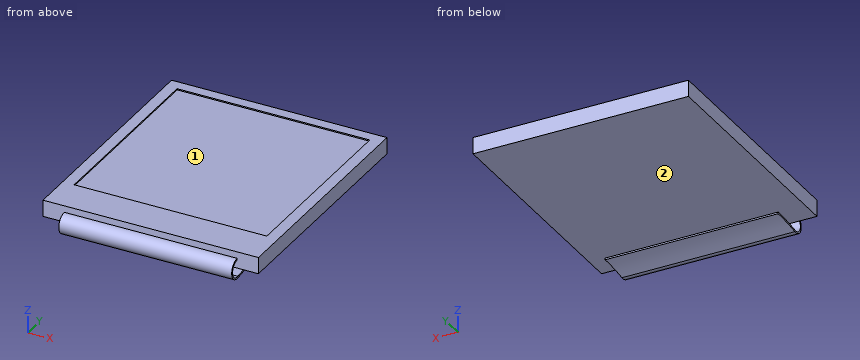
```python
from build123d import *

# Parameters (mm, degrees)
SKETCH001_W     = 26.16
SKETCH001_H     = 29.22
PAD001_DEPTH    = 2
SKETCH003_W     = 23.4
SKETCH003_H     = 23.4
POCKET001_DEPTH = 0.151
PAD002_DEPTH    = 10.5


with BuildPart() as part:
    # Sketch001 → Pad001 (new body)
    with BuildSketch(Plane.XY.offset(2.8)):
        Rectangle(SKETCH001_W, SKETCH001_H)
    extrude(amount=-PAD001_DEPTH)

    # Sketch003 → Pocket001 (cut, through all)
    with BuildSketch(Plane.XY.offset(2.65)):
        with Locations((0, 1.58)):
            Rectangle(SKETCH003_W, SKETCH003_H)
    extrude(amount=POCKET001_DEPTH, mode=Mode.SUBTRACT)

    # Sketch004 → Pad002 (join, symmetric)
    with BuildSketch(Plane.YZ):
        with BuildLine():
            ThreePointArc((-14.61, 2), (-15.856499, 0.656513), (-14.423549, -0.486016))
            ThreePointArc((-10.61, -0.2), (-12.52213, -0.271604), (-14.423549, -0.486016))
            Line((-10.61, 0), (-10.61, -0.2))
            ThreePointArc((-10.61, 0), (-12.537088, -0.072164), (-14.453381, -0.288254))
            ThreePointArc((-14.61, 1.8), (-15.657059, 0.671471), (-14.453381, -0.288254))
            Line((-14.61, 2), (-14.61, 1.8))
        make_face()
    extrude(amount=PAD002_DEPTH, both=True)


solid = part.part
```
Geometry: final body of the model. Coordinates: model frame, mm. Face numbers are marked on the shaded views. Coordinates: 2 decimals unless noted, no trailing zeros. Write each loop counter-clockwise with the first axis right and the second up, starting at its lowest first coordinate (ties: lowest second). Pieces come first, ordered by that corner, then holes. Notation, with made-up numbers: M -25.75,53.25 L 27.25,53.25 A21 ccw 27.25,76.25 Z; hole C 58.25,-28 d6. An arc over 180 degrees is marked long. Use CSV: the item, a comma, the result in double quotes. Start each with the question number.
1. Cut plane D-D on y = 8. Return the cut outline in (x, z), plus the area to 3 significant figures.
2. Mould query, pull axis X, two halves, no side actions, for the marked faces 1 and 2. Classes: pulls with the +X half, pulls with the -X half, needs draft (parallel to the pull), parting line crosses it, or undercut.
3. Cut plane C-C on x = -6.75. Return the cut outline in (y, z), plus the area to 3 significant figures.
4. Cut plane A-A on z = 1.35. Return the cut outline in (x, y), plus the area to 3 significant figures.
5. First-contact query: P1, Ø0.6, axis at x = 3.5, z = 2, coming from the -Y side; P2, Ø10, axis at x = -6.5, y = 1.5, coming from the -Z side; P3, Ø7, axis at x = -5.5, y = 5.5, coming from the +Z side; P4, Ø6, axis at x = -3, y = 10.5, coming from the +Z side. Flat tips, straight axial feed; report the tip coordinate or a pass-through.
6. Cut plane B-B on y = -12.5. Return the cut outline in (x, z), plus the area to 3 significant figures.
7. Ray query, probe 1 along Z at (x, y) = (-11.5, -13.5); probe 2 along Z at (x, y) = (10.75, 2.5); probe 3 along Y at (x, z) = (-11.25, 1.6). Return the intervals inside material, ascending.
Entries:
1,outline,"M -13.08,0.8 L 13.08,0.8 L 13.08,2.8 L 11.7,2.8 L 11.7,2.65 L -11.7,2.65 L -11.7,2.8 L -13.08,2.8 Z"
1,area,"48.8 mm²"
2,face 1,"undercut"
2,face 2,"needs draft"
3,outline,"M -14.61,0.8 L 14.61,0.8 L 14.61,2.8 L 13.28,2.8 L 13.28,2.65 L -10.12,2.65 L -10.12,2.8 L -14.61,2.8 L -14.61,2 A1.25 ccw long -14.42,-0.49 A25.57 cw -10.61,-0.2 L -10.61,0 A25.77 ccw -14.45,-0.29 A1.05 cw long -14.61,1.8 Z"
3,area,"56.5 mm²"
4,outline,"M -13.08,-14.61 L 13.08,-14.61 L 13.08,14.61 L -13.08,14.61 Z; M -10.5,-15.71 L 10.5,-15.71 L 10.5,-15.47 L -10.5,-15.47 Z"
4,area,"769 mm²"
5,P1,"y = -15.42"
5,P2,"z = 0.8"
5,P3,"z = 2.65"
5,P4,"z = 2.8"
6,outline,"M -13.08,0.8 L 13.08,0.8 L 13.08,2.8 L -13.08,2.8 Z; M -10.5,-0.27 L 10.5,-0.27 L 10.5,-0.07 L -10.5,-0.07 Z"
6,area,"56.5 mm²"
7,probe 1,"0.8 to 2.8"
7,probe 2,"0.8 to 2.65"
7,probe 3,"-14.61 to 14.61"
